Autodesk Fusion 360 part; units mm, degrees
sketch "Esquisse1" plane through (0, 0, 0) normal (0, 1, 0) x (1, 0, 0)
  line L0 (30, -20) -> (20, -20)
  line L1 (20, -20) -> (20, -10)
  line L2 (20, -10) -> (30, -10)
  line L3 (30, -10) -> (30, -20)
  circle A0 centre (25, -15) radius 1.25
  dimension "d1" = 10
  dimension "d2" = 10
  dimension "d22" = 2.5
extrude "Extrusion3" add sketch "Esquisse1" along normal blind 4
sketch "Esquisse3" plane through (0, 4, 0) normal (0, 1, 0) x (-1, 0, 0)
  circle A0 centre (-25, 15) radius 1.25
  line L0 (-30, 10) -> (-20, 10)
  line L1 (-20, 10) -> (-20, 20)
  line L2 (-20, 20) -> (-30, 20)
  line L3 (-30, 20) -> (-30, 10)
  line L4 (-30, 20) -> (-30, 17)
  line L5 (-30, 17) -> (-27.5, 17)
  line L6 (-27.5, 17) -> (-27.5, 15)
  line L7 (-27.5, 15) -> (-27, 15)
  line L8 (-25, 16.75) -> (-25, 17.5)
  line L9 (-25, 17.5) -> (-27, 17.5)
  line L10 (-27, 17.5) -> (-27, 20)
  line L11 (-27, 20) -> (-30, 20)
  line L12 (-30, 17) -> (-30, 20)
  line L13 (-26.75, 15) -> (-27.625, 15)
  line L14 (-25, 17.5) -> (-25, 17)
  line L15 (-25, 16.75) -> (-26.75, 16.75)
  line L16 (-26.75, 16.75) -> (-26.75, 15)
  line L17 (-27.5, 13) -> (-30, 13)
  line L18 (-30, 13) -> (-30, 10)
  line L19 (-30, 10) -> (-27, 10)
  line L20 (-27, 12.5) -> (-25, 12.5)
  line L21 (-25, 12.5) -> (-25, 13)
  line L22 (-27, 10) -> (-27, 12.5)
  line L23 (-25, 13.25) -> (-25, 12.375)
  line L24 (-26.75, 13.25) -> (-25, 13.25)
  line L25 (-26.75, 15) -> (-26.75, 13.25)
  line L26 (-26.75, 15) -> (-27.5, 15)
  line L27 (-27.5, 15) -> (-27.5, 13)
  line L28 (-23, 12.5) -> (-23, 10)
  line L29 (-23, 10) -> (-20, 10)
  line L30 (-20, 10) -> (-20, 13)
  line L31 (-22.5, 13) -> (-22.5, 15)
  line L32 (-22.5, 15) -> (-23, 15)
  line L33 (-20, 13) -> (-22.5, 13)
  line L34 (-23.25, 15) -> (-22.375, 15)
  line L35 (-23.25, 13.25) -> (-23.25, 15)
  line L36 (-25, 13.25) -> (-23.25, 13.25)
  line L37 (-25, 13.25) -> (-25, 12.5)
  line L38 (-25, 12.5) -> (-23, 12.5)
  line L39 (-22.5, 17) -> (-20, 17)
  line L40 (-20, 17) -> (-20, 20)
  line L41 (-20, 20) -> (-23, 20)
  line L42 (-23, 17.5) -> (-25, 17.5)
  line L43 (-25, 17.5) -> (-25, 17)
  line L44 (-23, 20) -> (-23, 17.5)
  line L45 (-25, 16.75) -> (-25, 17.625)
  line L46 (-23.25, 16.75) -> (-25, 16.75)
  line L47 (-23.25, 15) -> (-23.25, 16.75)
  line L48 (-23.25, 15) -> (-22.5, 15)
  line L49 (-22.5, 15) -> (-22.5, 17)
  dimension "d19" = 2.5
  dimension "d20" = 2.5
  dimension "d21" = 2.5
  dimension "d25" = 360
  dimension "d27" = 0.75
  dimension "d28" = 0.75
  dimension "d36" = 4
  dimension "d37" = 3
  dimension "d38" = 3
  dimension "d39" = 3.5
extrude "Extrusion6" add sketch "Esquisse3" along normal blind 46 contours L0 L3 L7 L13 L17 L18 L19 L20 L21 L22 L23 L24 L25 L26 L27 L37 | L0 L1 L21 L23 L28 L29 L30 L31 L32 L33 L34 L35 L36 L37 L38 L48 | L2 L3 L4 L5 L6 L7 L8 L9 L10 L11 L12 L13 L14 L15 L16 L26 L43 L45 | L1 L2 L8 L14 L32 L34 L39 L40 L41 L42 L43 L44 L45 L46 L47 L48 L49
fillet "Congé2" radius 1 4 edges at (23.25, 27, 13.25) (26.75, 27, 13.25) (26.75, 27, 16.75) (23.25, 27, 16.75)
sketch "Esquisse4" plane through (0, 0, 0) normal (0, -1, 0) x (1, 0, 0)
  circle A0 centre (25, 15) radius 1.25
  line L0 (20, 10) -> (30, 10)
  line L1 (30, 10) -> (30, 20)
  line L2 (30, 20) -> (20, 20)
  line L3 (20, 20) -> (20, 10)
  line L4 (23.5266, 12.5173) -> (26.4134, 12.4827)
  line L5 (26.4134, 12.4827) -> (27.8868, 14.9654)
  line L6 (27.8868, 14.9654) -> (26.4734, 17.4827)
  line L7 (26.4734, 17.4827) -> (23.5866, 17.5173)
  line L8 (23.5866, 17.5173) -> (20, 17.5173)
  line L9 (23.5266, 12.5173) -> (20, 12.5173)
  point P0 (25, 15)
extrude "Extrusion7" cut sketch "Esquisse4" against normal blind 2 contours L3 L4 L5 L6 L7 L8 L9
Read the model definition and answer for the solid it produces. Units are mm, in the model's axes. A direction names the side the tool comes from. Round coordinates to 2 decimals unless told otherwise and drop trailing zeros. Write each loop counter-clockwise with the first axis right and the second up, starting at its lowest first coordinate (ties: lowest second). Pieces come first, ordered by that corner, then holes. Notation, with made-up numbers: (84, 14) -> (105, 14) arc R6 ccw to (105, 21) -> close; hole circle Ø8 at (-22, 25.5). An arc over 180 degrees is marked (long way). Answer in a Markdown table with one row per item. Add a question column.
1) Given P1, Ø1, axis at x = 25, y = 37.5, coming from the +Z side; P2, Ø2, axis at y = 18.5, z = 15.5, coming from the -X side; P3, Ø1.2, axis at y = 33.5, z = 15, coming from the +X side; P4, Ø1, axis at x = 24.5, z = 14.5, coming from the +Y side, each flat-ended and moving along its own axis, determine where each tip first touches the part or whether it passes through.
2) Find section B-B, the plane x = 25. Determine the outline of the cut face in (y, z), and give its area (3 significant figures).
3) Find section C-C, the plane y = 42. Determine the outline of the cut face in (x, z).
4) Find section A-A, the plane z = 18.5. Determine the outline of the cut face in (x, y).
5) Determine the mould class of faces 4 (the face through (25, 27, 16.75)), 5 (the face through (27, 27, 19)) for opening direction Z: pulls with the +Z half, pulls with the -Z half, needs draft (parallel to the pull), parting line crosses it, or undercut.
6) Consider line 1 (Z direction, x = 28.25, y = 16); line 2 (X direction, y = 22, z = 19); line 3 (X direction, y = 2.8, z = 15). Determine where each line is inside the solid, lowest interval first.
7) Which of the six approach directions +Z, -Z, +X, -X, +Y, -Y give full straight-line access (tool end or side, diameter ignored) to faces 1 (the face through (27.19, 0.99, 16.21)), 2 (the face through (23.25, 27, 15)), 3 (the face through (29, 27, 13))?
Findings below:
| question | item | result |
|---|---|---|
| 1 | P1 | z = 17.5 |
| 1 | P2 | x = 22.5 |
| 1 | P3 | x = 27.5 |
| 1 | P4 | through |
| 2 | outline | (0, 10) -> (4, 10) -> (4, 12.5) -> (50, 12.5) -> (50, 13.25) -> (4, 13.25) -> (4, 13.75) -> (2, 13.75) -> (2, 12.5) -> (0, 12.5) -> close; (0, 17.5) -> (2, 17.5) -> (2, 16.25) -> (4, 16.25) -> (4, 16.75) -> (50, 16.75) -> (50, 17.5) -> (4, 17.5) -> (4, 20) -> (0, 20) -> close |
| 2 | area | 94.0 mm² |
| 3 | outline | (20, 10) -> (23, 10) -> (23, 12.5) -> (27, 12.5) -> (27, 10) -> (30, 10) -> (30, 13) -> (27.5, 13) -> (27.5, 17) -> (30, 17) -> (30, 20) -> (27, 20) -> (27, 17.5) -> (23, 17.5) -> (23, 20) -> (20, 20) -> (20, 17) -> (22.5, 17) -> (22.5, 13) -> (20, 13) -> close; hole (23.25, 14.25) arc R1 ccw to (24.25, 13.25) -> (25.75, 13.25) arc R1 ccw to (26.75, 14.25) -> (26.75, 15.75) arc R1 ccw to (25.75, 16.75) -> (24.25, 16.75) arc R1 ccw to (23.25, 15.75) -> close |
| 4 | outline | (20, 0) -> (30, 0) -> (30, 50) -> (27, 50) -> (27, 4) -> (23, 4) -> (23, 50) -> (20, 50) -> close |
| 5 | face 4 | undercut |
| 5 | face 5 | needs draft |
| 6 | line 1 | 10 to 13, 17 to 20 |
| 6 | line 2 | 20 to 23, 27 to 30 |
| 6 | line 3 | 20 to 23.75, 26.25 to 30 |
| 7 | face 1 | -X, -Y |
| 7 | face 2 | +Y |
| 7 | face 3 | +X, +Y |
